Source: CAD feature listing. Evaluate the final solid. Frame: model axes, mm. A direction names the side the tool comes from. Round coordinates to 2 decimals unless told otherwise and drop trailing zeros. Loops run counter-clockwise (first coordinate to the right, second up) from the corner with the lowest first, then second, coordinate; pieces in that order, holes last.
Item 1: Ray query, L1, parallel to Z at x = -4.5, y = -3.5; L2, parallel to Y at x = -17, z = 2230.5; L3, parallel to X at y = 211, z = 2118. Return the intervals inside material, ascending.
Item 2: Section query B-B on y = 256. Return loops of the section in (x, z).
Item 3: Access query for faces 1 (the cylindrical face through (-43.67, -306.81, 1183.29)), 2 (the flat face through (-25, 253, 1183)). Directions: +Z, -Z, +X, -X, +Y, -Y. A direction counts if a zero-diameter tool reaches every point of the face in a straight line with its end or side. Return the directions, or none.
Item 4: Section query A-A on z = 2044.5. Return loops of the section in (x, y), then the cut area to 3 significant figures.
```python
from build123d import *

# Parameters (mm, degrees)
F1_DEPTH = 2400
F2_R     = 6.5


with BuildPart() as f1:
    # F0 (on Top) → F1 (new body)
    with BuildSketch(Plane.XY):
        with BuildLine():
            Line((-20, 301.836108), (-25, 301.836108))
            Line((-25, 301.836108), (-25, 201.836108))
            Line((-25, 201.836108), (-50, 201.836108))
            Line((-50, 201.836108), (-50, -258.163892))
            ThreePointArc((-50, -258.163892), (-43.491581, -307.48237), (-24.411949, -353.424066))
            ThreePointArc((-24.411949, -353.424066), (-20.9355, -356.89407), (-16.19059, -358.163892))
            Line((-16.19059, -358.163892), (-6.5, -358.163892))
            ThreePointArc((-6.5, -358.163892), (-1.903806, -356.260086), (0, -351.663892))
            Line((0, -351.663892), (0, 281.836108))
            ThreePointArc((0, 281.836108), (-5.857864, 295.978244), (-20, 301.836108))
        make_face()
    extrude(amount=F1_DEPTH)

    # F2
    f2_edges = [f1.edges().sort_by_distance(p)[0] for p in [
        (-50, -28.163892, 2400),
        (-50, -28.163892, 0),
    ]]
    fillet(f2_edges, radius=F2_R)


solid = f1.part
```
Data:
1. L1: z = 0.32 to 2399.68
1. L2: y = -358.13 to 301.61
1. L3: x = -25 to 0
2. outline: (-25, 0) - (-6.5, 0) arc R6.5 ccw to (0, 6.5) - (0, 2393.5) arc R6.5 ccw to (-6.5, 2400) - (-25, 2400) - close
3. face 1: +Z, -Z, -X, -Y
3. face 2: +Z, -Z, -X, +Y
4. outline: (-50, -258.16) arc R190.11 ccw to (-24.41, -353.42) arc R9.5 ccw to (-16.19, -358.16) - (-6.5, -358.16) arc R6.5 ccw to (0, -351.66) - (0, 281.84) arc R20 ccw to (-20, 301.84) - (-25, 301.84) - (-25, 201.84) - (-50, 201.84) - close
4. area: 29,500 mm2
